from build123d import *

# Parameters (mm, degrees)
CROQUIS1_W                   = 40
CROQUIS1_H                   = 80
CROQUIS1_R                   = 3.25
SALIENTE_EXTRUIR1_DEPTH      = 7
CROQUIS2_R                   = 6.5
CORTAR_EXTRUIR1_DEPTH        = 5
CROQUIS3_R                   = 6
CORTAR_EXTRUIR2_DEPTH        = 0.5
REDONDEO2_R                  = 3
SALIENTE_EXTRUIR2_DEPTH      = 5
TALADROAVANZADO1_OUTLINE_R   = 1.2
TALADROAVANZADO1_DEPTH       = 1
TALADROAVANZADO1_DRAFT       = -45
TALADROAVANZADO1_2_OUTLINE_R = 1.2
TALADROAVANZADO1_2_DEPTH     = 1
TALADROAVANZADO1_2_DRAFT     = -45
CORTAR_EXTRUIR3_START        = 1
CROQUIS8_R                   = 1.2
CORTAR_EXTRUIR3_DEPTH        = 83.124903698


# Read off the part's stored shape, not the designer's step: TaladroAvanzado1
with BuildPart() as part:
    # Croquis1 → Saliente-Extruir1 (new body)
    with BuildSketch(Plane.XY):
        Rectangle(CROQUIS1_W, CROQUIS1_H)
        with Locations((-5, 20)):
            Circle(CROQUIS1_R, mode=Mode.SUBTRACT)
    extrude(amount=SALIENTE_EXTRUIR1_DEPTH)

    # Croquis2 → Cortar-Extruir1 (cut)
    with BuildSketch(Plane(origin=(0, 0, 0), x_dir=(-1, 0, 0), z_dir=(0, 0, -1))):
        with Locations((5, 20)):
            Circle(CROQUIS2_R)
    extrude(amount=-CORTAR_EXTRUIR1_DEPTH, mode=Mode.SUBTRACT)

    # Croquis3 → Cortar-Extruir2 (cut)
    with BuildSketch(Plane(origin=(0, 0, 5), x_dir=(-1, 0, 0), z_dir=(0, 0, -1))):
        with Locations((5, 20)):
            Circle(CROQUIS3_R)
    extrude(amount=-CORTAR_EXTRUIR2_DEPTH, mode=Mode.SUBTRACT)

    # Redondeo2
    redondeo2_edges = [part.edges().sort_by_distance(p)[0] for p in [
        (-20, 40, 3.5),
        (20, 40, 3.5),
        (20, 0, 7),
        (0, 40, 7),
        (-20, 0, 7),
        (-20, 0, 0),
        (0, 40, 0),
        (20, 0, 0),
    ]]
    fillet(redondeo2_edges, radius=REDONDEO2_R)

    # Croquis4 → Saliente-Extruir2 (add)
    with BuildSketch(Plane.XZ.offset(40)):
        with BuildLine():
            Line((-17, 7), (-24, 7))
            ThreePointArc((-24, 7), (-27.5, 3.5), (-24, 0))
            Line((-24, 0), (-17, 0))
            Line((-17, 0), (-17, 7))
        make_face()
        with BuildLine():
            Line((17, 7), (24, 7))
            ThreePointArc((24, 7), (27.5, 3.5), (24, 0))
            Line((24, 0), (17, 0))
            Line((17, 0), (17, 7))
        make_face()
    extrude(amount=-SALIENTE_EXTRUIR2_DEPTH)


with BuildPart() as taladroavanzado1_tool:
    # TaladroAvanzado1 outline → TaladroAvanzado1 (with draft: the straight prism first)
    with BuildSketch(Plane(origin=(0, -36, 0), x_dir=(1, 0, 0), z_dir=(0, 1, 0))):
        with Locations((24, -3.5)):
            Circle(TALADROAVANZADO1_OUTLINE_R)
    extrude(amount=TALADROAVANZADO1_DEPTH)
    # TaladroAvanzado1: the draft: its side faces are tilted about the plane it starts from
    taladroavanzado1_sides = [taladroavanzado1_tool.faces().sort_by_distance(p)[0] for p in [
        (22.8, -35.5, 3.5),
    ]]
    draft(taladroavanzado1_sides, Plane(origin=(0, -36, 0), x_dir=(1, 0, 0), z_dir=(0, 1, 0)), TALADROAVANZADO1_DRAFT)


with BuildPart() as part_1:
    add(part.part)

    # TaladroAvanzado1: cut by taladroavanzado1_tool
    add(taladroavanzado1_tool.part, mode=Mode.SUBTRACT)


with BuildPart() as taladroavanzado1_2_tool:
    # TaladroAvanzado1 2 outline → TaladroAvanzado1 2 (with draft: the straight prism first)
    with BuildSketch(Plane(origin=(0, -36, 0), x_dir=(1, 0, 0), z_dir=(0, 1, 0))):
        with Locations((-24, -3.5)):
            Circle(TALADROAVANZADO1_2_OUTLINE_R)
    extrude(amount=TALADROAVANZADO1_2_DEPTH)
    # TaladroAvanzado1 2: the draft: its side faces are tilted about the plane it starts from
    taladroavanzado1_2_sides = [taladroavanzado1_2_tool.faces().sort_by_distance(p)[0] for p in [
        (-25.2, -35.5, 3.5),
    ]]
    draft(taladroavanzado1_2_sides, Plane(origin=(0, -36, 0), x_dir=(1, 0, 0), z_dir=(0, 1, 0)), TALADROAVANZADO1_2_DRAFT)


with BuildPart() as part_2:
    add(part_1.part)

    # TaladroAvanzado1 2: cut by taladroavanzado1_2_tool
    add(taladroavanzado1_2_tool.part, mode=Mode.SUBTRACT)

    # Croquis8 → Cortar-Extruir3 (cut, through all)
    with BuildSketch(Plane(origin=(0, -36, 0), x_dir=(1, 0, 0), z_dir=(0, 1, 0)).offset(CORTAR_EXTRUIR3_START)):
        with Locations(Location((24, -3.5, 0), (0, 0, 90))):
            Circle(CROQUIS8_R)
        with Locations(Location((-24, -3.5, 0), (0, 0, 90))):
            Circle(CROQUIS8_R)
    extrude(amount=-CORTAR_EXTRUIR3_DEPTH, mode=Mode.SUBTRACT)


solid = part_2.part
Model file for the job. Use its own axes, mm. A direction names the side the tool comes from. Coordinates: 2 decimals unless noted, no trailing zeros. Order: outer loops, then holes, each group sorted by start corner. A loop starts at its lowest first (then second) coordinate and runs counter-clockwise, first axis right, second up. Notation, with made-up numbers: (-26.75, 22.5) -> (-19.75, 22.5) arc R26 ccw to (-19.75, 51.5) -> close; hole circle Ø6 at (16, -14.5). An arc over 180 degrees is marked (long way). Return JSON: item names as keys, results as strings. Group by question number.
Item 1: Saw through at A-A on y = 20. Write the cut outline in (x, z), then the cut area to 3 significant figures.
Item 2: Wall check: line 1 along Y through (x, z) = (-5, 3); line 2 along Z through (x, y) = (-24, -36.9); line 3 along X through (y, z) = (17, 3.5). Give the ranges that are in metal, low to high. Write a range as [from, to].
Item 3: Tool access for faces 5 (the cylindrical face through (0.994, 20.264, 5.246)), 6 (the cylindrical face through (-19.14, 1.5, 6.1)), 7 (the cylindrical face through (-19.14, 1.5, 0.9)): list every direction of +Z, -Z, +X, -X, +Y, -Y with a clear straight run to the whole face (end or side of a thin tool).
Item 4: Flat gauge pins, fed straight in: P1, Ø5, axis at x = -17, y = 20.5, coming from the -Z side; P2, Ø3, axis at x = 19.5, z = 1, coming from the +Y side; P3, Ø10.5, axis at x = -5, y = 20, coming from the -Z side; P4, Ø3.5, axis at x = 23, z = 2, coming from the +Y side. Where does each tip first touch, or does it go through?
Item 5: Saw through at C-C on x = -19. Write the cut outline in (y, z).
Item 6: Saw through at B-B on y = -31. Write the cut outline in (x, z).
Item 7: Pull direction X, two halves, no side cores. Call faces 1 (the cylindrical face through (-5.705, 16.827, 6.24)), 2 (the cylindrical face through (-27.5, -37.5, 3.6)), 3 (the flat face through (0, -2, 0)), 4 (the flat face through (-8, 17, 5.5)): pulls with the +X half, pulls with the -X half, needs draft (parallel to the pull), parting line crosses it, or undercut.
Values found:
{
 "1": {"outline": "(-20, 3) arc R3 ccw to (-17, 0) -> (-11.5, 0) -> (-11.5, 5) -> (-11, 5) -> (-11, 5.5) -> (-8.25, 5.5) -> (-8.25, 7) -> (-17, 7) arc R3 ccw to (-20, 4) -> close; (-1.75, 5.5) -> (1, 5.5) -> (1, 5) -> (1.5, 5) -> (1.5, 0) -> (17, 0) arc R3 ccw to (20, 3) -> (20, 4) arc R3 ccw to (17, 7) -> (-1.75, 7) -> close", "area": "192 mm2"},
 "2": {"line 1": "y = [-40, 13.5], [26.5, 40]", "line 2": "z = [0, 2.3], [4.7, 7]", "line 3": "x = [-20, -10.77], [0.77, 20]"},
 "3": {"face 5": "-Z", "face 6": "+Z, -X, +Y", "face 7": "-Z, -X, +Y"},
 "4": {"P1": "stops at z = 0", "P2": "stops at y = 39.47", "P3": "stops at z = 5.5", "P4": "stops at y = -35"},
 "5": {"outline": "(-40, 0) -> (-35, 0) -> (-35, 0.76) -> (37, 0.76) arc R2.24 ccw to (39.24, 3) -> (39.24, 4) arc R2.24 ccw to (37, 6.24) -> (-35, 6.24) -> (-35, 7) -> (-40, 7) -> close"},
 "6": {"outline": "(-20, 3) arc R3 ccw to (-17, 0) -> (17, 0) arc R3 ccw to (20, 3) -> (20, 4) arc R3 ccw to (17, 7) -> (-17, 7) arc R3 ccw to (-20, 4) -> close"},
 "7": {"face 1": "undercut", "face 2": "pulls with the -X half", "face 3": "needs draft", "face 4": "undercut"}
}
